Here's how the part is built. I have some questions about the finished solid (model axes, mm). A direction names the side the tool comes from. Round coordinates to 2 decimals unless told otherwise and drop trailing zeros. Loops run counter-clockwise (first coordinate to the right, second up) from the corner with the lowest first, then second, coordinate; pieces in that order, holes last. Notation, with made-up numbers: M 67,-40 L 73,-40 A27 cw 73,-23 Z; hole C 59,-11.75 d7. An arc over 180 degrees is marked long. Write each question's results on one line, items separated by ' | '. Start each with the question number.
```python
from build123d import *

# Parameters (mm, degrees)
BOSS_EXTRUDE1_DEPTH = 5
BOSS_EXTRUDE4_DEPTH = 20
BOSS_EXTRUDE5_DEPTH = 20


with BuildPart() as part:
    # Sketch1 → Boss-Extrude1 (new body)
    with BuildSketch(Plane(origin=(0, 0, 0), x_dir=(0, 1, 0), z_dir=(0, 0, 1))):
        Polygon((-65.650485437, 9.713592233), (-65.650485437, -13.286407767), (-48.650485437, -13.286407767), (-48.650485437, -76.836407767), (151.449514563, -76.836407767), (151.449514563, -26.836407767), (191.449514563, -26.836407767), (191.449514563, 23.263592233), (151.449514563, 23.263592233), (151.449514563, 73.263592233), (-48.650485437, 73.263592233), (-48.650485437, 9.713592233), align=None)
    extrude(amount=BOSS_EXTRUDE1_DEPTH)

    # Sketch7 → Boss-Extrude4 (add)
    with BuildSketch(Plane.XY.offset(5)):
        Polygon((-23.263592233, 151.449514563), (-73.263592233, 151.449514563), (-73.263592233, -48.650485437), (-9.713592233, -48.650485437), (-9.713592233, -43.650485437), (-68.263592233, -43.650485437), (-68.263592233, 146.449514563), (-23.263592233, 146.449514563), align=None)
    extrude(amount=BOSS_EXTRUDE4_DEPTH)

    # Sketch9 → Boss-Extrude5 (add)
    with BuildSketch(Plane.XY.offset(5)):
        Polygon((26.836407767, 151.449514563), (76.836407767, 151.449514563), (76.836407767, -48.650485437), (13.286407767, -48.650485437), (13.286407767, -43.650485437), (71.836407767, -43.650485437), (71.836407767, 146.449514563), (26.836407767, 146.449514563), align=None)
    extrude(amount=BOSS_EXTRUDE5_DEPTH)


solid = part.part
```
Item 1: If we section it at C-C on x = -48: Please give me the cut outline in (y, z), and give its area (3 significant figures).
Item 2: If we mould it in two halves opening along Y, with no side actions, what happens to faces 6 (the face through (51, 151.45, 12)), 7 (the face through (26.836, 149, 15)), 8 (the face through (71.836, 50, 15))? For each: released by +Y, released by -Y, zero draft, split by the parting line, or undercut.
Item 3: If we section it at D-D on y = 164.5: Please give me the cut outline in (x, z), and give its area (4 significant figures).
Item 4: Which directions (+Z, -Z, +X, -X, +Y, -Y) give clear straight access to the entire face, cutting with the end or side of a thin tool? Please do faces 1 (the face through (-42, -48.65, 12)), 2 (the face through (46, -48.65, 12)), 3 (the face through (13.286, -46, 15)), 4 (the face through (26.836, 171, 2)), 5 (the face through (42, -43.65, 15)).
Item 5: I'm going to push flat-ended pins straight in: pin 1 (3 mm diameter, centred on x = -57, z = 11, fed in from -Y); pin 2 (2.5 mm diameter, centred on y = -59.5, z = 2, fed in from +X); pin 3 (5 mm diameter, centred on x = -50, z = 17, fed in from +Y). Where does each tip first touch, or does it pass through?
Item 6: If we section it at A-A on z = 13: Please give me the cut outline in (x, y), and give its area (3 significant figures).
Item 7: If we section it at B-B on y = 102.5: Please give me the cut outline in (x, z), and give its area (4 significant figures).
Item 8: I need wall thicknesses on L1, parallel to X at y = 125.5, z = 13.75; L2, parallel to Y at x = 59, z = 14.5; L3, parallel to Y at x = -34.5, z = 4. Which ranges of each line are inside material? Lowest first, please.
Numbers:
1) outline: M -48.65,0 L 151.45,0 L 151.45,25 L 146.45,25 L 146.45,5 L -43.65,5 L -43.65,25 L -48.65,25 Z | area: 1,200 mm²
2) face 6: released by +Y | face 7: zero draft | face 8: undercut
3) outline: M -23.26,0 L 26.84,0 L 26.84,5 L -23.26,5 Z | area: 250.5 mm²
4) face 1: +Z, -Z, -X, -Y | face 2: +Z, -Z, +X, -Y | face 3: +Z, +Y, -Y | face 4: +Z, -Z, +X, +Y | face 5: +Z
5) pin 1: y = -48.65 | pin 2: x = 13.29 | pin 3: y = 151.45
6) outline: M -73.26,-48.65 L -9.71,-48.65 L -9.71,-43.65 L -68.26,-43.65 L -68.26,146.45 L -23.26,146.45 L -23.26,151.45 L -73.26,151.45 Z; M 13.29,-48.65 L 76.84,-48.65 L 76.84,151.45 L 26.84,151.45 L 26.84,146.45 L 71.84,146.45 L 71.84,-43.65 L 13.29,-43.65 Z | area: 3,040 mm²
7) outline: M -73.26,0 L 76.84,0 L 76.84,25 L 71.84,25 L 71.84,5 L -68.26,5 L -68.26,25 L -73.26,25 Z | area: 950.5 mm²
8) L1: -73.26 to -68.26, 71.84 to 76.84 | L2: -48.65 to -43.65, 146.45 to 151.45 | L3: -48.65 to 151.45
